from build123d import *

# Parameters (mm, degrees)
F0_W     = 150
F0_H     = 50
F1_DEPTH = 25
F3_DEPTH = 1
F4_R     = 10
F5_ANGLE = -180


with BuildPart() as f1:
    # F0 (on Top) → F1 (new body)
    with BuildSketch(Plane.XY):
        Rectangle(F0_W, F0_H)
    extrude(amount=F1_DEPTH)

    # F2 (on face) → F3 (join)
    with BuildSketch(Plane.XY.offset(25)):
        Polygon((-20.35143, -13.440839), (-16.17611, -13.440839), (-31.457786, 17.728945), (-44.317774, -13.440839), (-40.142454, -13.440839), (-36.851476, -4.382354), (-24.560086, -4.382354), align=None)
        Polygon((-35.80012, -1.488477), (-31.457786, 10.463886), (-25.904608, -1.488477), align=None, mode=Mode.SUBTRACT)
        Polygon((10.236647, 14.533813), (10.236647, 17.707057), (-6.715158, 17.707057), (-9.637882, 17.707057), (7.647947, -11.186166), (-7.049183, -11.186166), (-7.049183, -13.440839), (12.658333, -13.440839), (-4.741451, 14.533813), align=None)
        with BuildLine():
            Line((30.189158, -5.461854), (30.189158, -14.399434))
            Line((30.189158, -14.399434), (31.969018, -14.419133))
            Line((31.969018, -14.419133), (31.969018, 17.378626))
            Line((31.969018, 17.378626), (30.189158, 17.378626))
            ThreePointArc((30.189158, 17.378626), (20.49841, 9.434111), (30.189158, 1.489596))
            Line((30.189158, 1.489596), (20.0599, -13.803595))
            Line((20.0599, -13.803595), (24.429381, -13.803595))
            Line((24.429381, -13.803595), (30.189158, -5.461854))
        make_face()
        with BuildLine():
            ThreePointArc((30.189158, 3.674338), (24.891917, 8.987233), (30.189158, 14.300127))
            Line((30.189158, 14.300127), (30.189158, 3.674338))
        make_face(mode=Mode.SUBTRACT)
        Polygon((57.79634, 16.385563), (38.729511, 16.385563), (38.729511, 12.214691), (52.63241, 12.214691), (52.63241, 5.461854), (39.325345, 5.461854), (39.325345, 0), (52.83102, 0), (52.83102, -9.036886), (39.921183, -9.036886), (39.921183, -14.399434), (57.79634, -14.399434), align=None)
    extrude(amount=F3_DEPTH)

    # F4 (on face) → F5 (revolve)
    with BuildSketch(Plane(origin=(0, 0, 0), x_dir=(1, 0, 0), z_dir=(0, 0, -1))):
        with Locations((32.374486, 0)):
            Circle(F4_R)
    revolve(axis=Axis((0, -0.202699, 0), (0, -1, 0)), revolution_arc=F5_ANGLE)


solid = f1.part
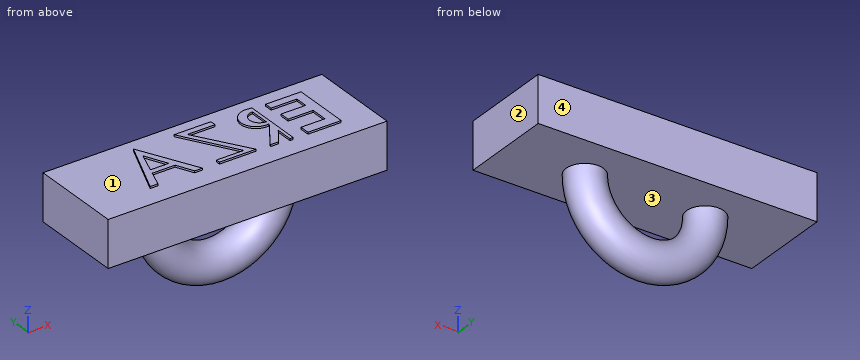
Work out the finished part from the listing and answer in its coordinate system (mm). Face numbers are marked on the shaded views. Give positions to 0.01 mm unless a question says otherwise; leave off trailing zeros. Write each loop counter-clockwise with the first axis right and the second up, starting at its lowest first coordinate (ties: lowest second). Pieces come first, ordered by that corner, then holes. Notation, with made-up numbers: (58.25, 31.25) - (114.25, 31.25) arc R29 cw to (114.25, 59.25) - close; hole circle Ø4 at (56.25, 37.25). An arc over 180 degrees is marked (long way). One line per item, written item: value. Start each with the question number.
1. Given pin 1 (5 mm diameter, centred on x = -8.5, y = -15.5, fed in from -Z); pin 2 (0.8 mm diameter, centred on x = 49, z = 25.5, fed in from +Y); pin 3 (0.8 mm diameter, centred on x = 23, z = 25.5, fed in from -Y), each flat-ended and moving along its own axis, determine where each tip first touches the part or whether it passes through.
2. Consider probe 1 along Z at (x, y) = (64.5, -21.5); probe 2 along Z at (x, y) = (10.5, 0.5); probe 3 along Z at (x, y) = (-9.5, -9). Determine where each line is inside the solid, lowest interval first.
3. Find section A-A (x = 48.5). Write down the section's boundary in (y, z), then the cut area to 3 significant figures.
4. Find section B-B (y = -18). Write down the section's boundary in (x, z), then the cut area to 3 significant figures.
5. For a pull along X with two mould halves and no side action, classify the marked faces 1, 2, 3 and 4 as +X half, -X half, draft (parallel to the pull), parting line (faces both ways), or undercut.
Geometry results:
1. pin 1: z = 0
1. pin 2: y = 16.39
1. pin 3: y = -13.8
2. probe 1: 0 to 25
2. probe 2: -41.04 to -19.77, 0 to 25
2. probe 3: -35.48 to -26.36, 0 to 25
3. outline: (-25, 0) - (25, 0) - (25, 25) - (16.39, 25) - (16.39, 26) - (12.21, 26) - (12.21, 25) - (5.46, 25) - (5.46, 26) - (0, 26) - (0, 25) - (-9.04, 25) - (-9.04, 26) - (-14.4, 26) - (-14.4, 25) - (-25, 25) - close
3. area: 1,260 mm2
4. outline: (-75, 0) - (75, 0) - (75, 25) - (-75, 25) - close
4. area: 3,750 mm2
5. face 1: undercut
5. face 2: +X half
5. face 3: undercut
5. face 4: draft
